Job drawing, mm, ordinate dimensions from the low corner. One solid piece. Round coordinates to 2 decimals unless told otherwise and drop trailing zeros. Write each loop counter-clockwise with the first axis right and the second up, starting at its lowest first coordinate (ties: lowest second). Pieces come first, ordered by that corner, then holes. Notation, with made-up numbers: M 12.5,78 L 39.5,78 A25 cw 39.5,95 Z; hole C 21.5,38 d7. An arc over 180 degrees is marked long. One line per item, written item: value. Start each with the question number.
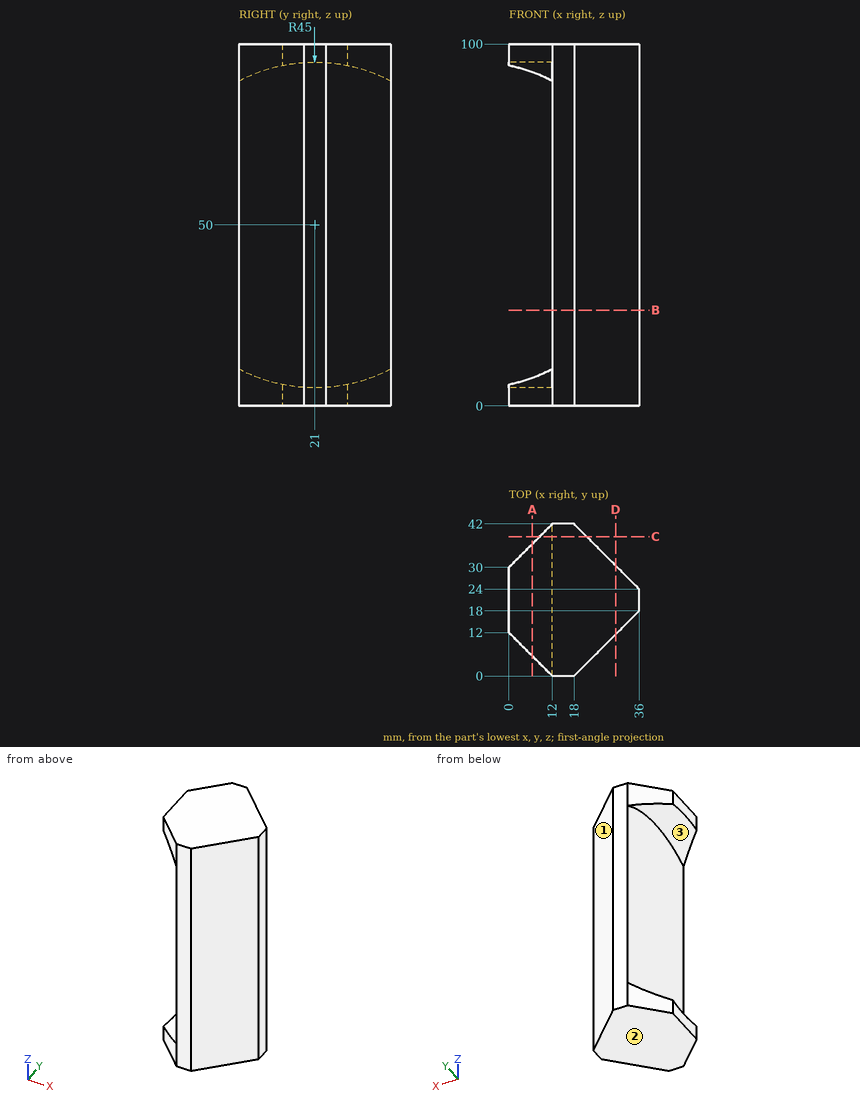
Item 1: Cut at D-D, the plane x = 29.5. Write the cut outline in (y, z), plus the area to 3 significant figures.
Item 2: Two-plate mould, pull along Z, no slides. Class the marked faces 1, 2 and 3: pulls with the +Z half, pulls with the -Z half, needs draft (parallel to the pull), parting line crosses it, or undercut.
Item 3: Drill centre lines: line 1 (Z direction, x = 4, y = 21); line 2 (X direction, y = 6, z = 36.5); line 3 (X direction, y = 22, z = 12.5). Where is each one in solid material? Low to high.
Item 4: Cut at C-C, the plane y = 38.5. Write the cut outline in (x, z).
Item 5: Drop flat-ended pins along their axis: pin 1 (4 mm diameter, centred on x = 20.5, z = 83.5, fed in from +Y); pin 2 (1 mm diameter, centred on y = 28, z = 78, fed in from -X); pin 3 (3 mm diameter, centred on x = 8.5, z = 12, fed in from +Y). Give the stop position or say it passes through.
Item 6: Cut at B-B, the plane z = 26.5. Write the cut outline in (x, y), plus the area to 3 significant figures.
Item 7: Cut at A-A, the plane x = 6.5. Write the cut outline in (y, z), plus the area to 3 significant figures.
Computed values:
1. outline: M 11.5,0 L 30.5,0 L 30.5,100 L 11.5,100 Z
1. area: 1,900 mm2
2. face 1: needs draft
2. face 2: pulls with the -Z half
2. face 3: undercut
3. line 1: z = 0 to 5, 95 to 100
3. line 2: x = 12 to 24
3. line 3: x = 12 to 36
4. outline: M 8.5,0 L 21.5,0 L 21.5,100 L 8.5,100 L 8.5,91.46 L 12,91.46 L 12,8.54 L 8.5,8.54 Z
5. pin 1: stops at y = 41.5
5. pin 2: stops at x = 12
5. pin 3: passes through
6. outline: M 12,0 L 18,0 L 36,18 L 36,24 L 18,42 L 12,42 Z
6. area: 684 mm2
7. outline: M 5.5,0 L 36.5,0 L 36.5,7.75 A45 cw 5.5,7.75 Z; M 5.5,92.25 A45 cw 36.5,92.25 L 36.5,100 L 5.5,100 Z
7. area: 366 mm2
